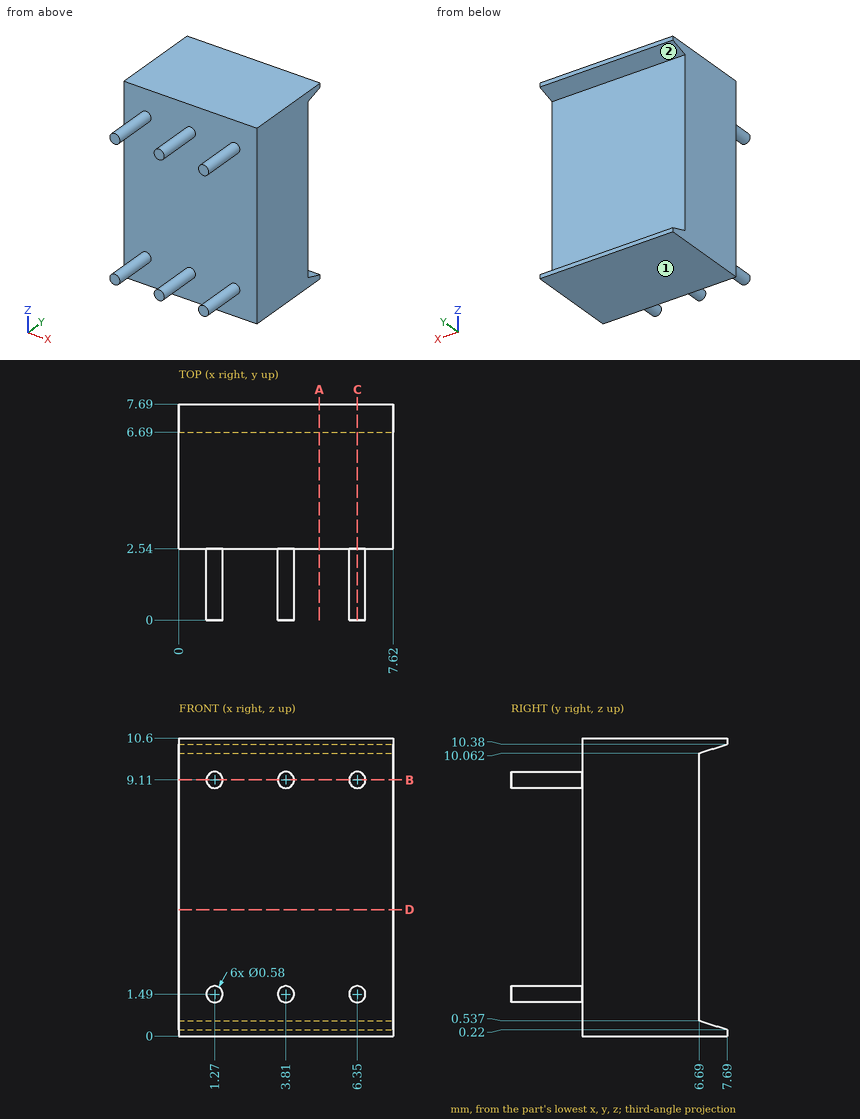
Part print with two shaded views. Sizes in mm from the minimum x, y, z corner. A direction names the side the tool comes from. Round coordinates to 2 decimals unless told otherwise and drop trailing zeros. Loops run counter-clockwise (first coordinate to the right, second up) from the corner with the lowest first, then second, coordinate; pieces in that order, holes last.
1. Slice it at A-A (x = 5). Give the cut face in (y, z).
Solutions:
outline: (2.54, 0) - (7.69, 0) - (7.69, 0.22) - (6.69, 0.54) - (6.69, 10.06) - (7.69, 10.38) - (7.69, 10.6) - (2.54, 10.6) - close
2. Drill centre lines: line 1 along Y through (x, z) = (7, 9.25); line 2 along Z through (x, y) = (4, 1.75); line 3 along Z through (x, y) = (5.75, 6.75). Where is each one in solid material? Low to high.
Solutions:
line 1: y = 2.54 to 6.69
line 2: z = 1.27 to 1.71, 8.89 to 9.33
line 3: z = 0 to 0.52, 10.08 to 10.6
3. Flat gauge pins, fed straight in: pin 1 (1 mm diameter, centred on x = 3.5, z = 8.5, fed in from -Y); pin 2 (4 mm diameter, centred on x = 5.5, z = 4.5, fed in from +Y); pin 3 (4 mm diameter, centred on x = 6, z = 4, fed in from -Y). Where does each tip first touch, or does it go through?
Solutions:
pin 1: stops at y = 0
pin 2: stops at y = 6.69
pin 3: stops at y = 2.54
4. Slice it at D-D (z = 4.5). Give the cut face in (x, y).
Solutions:
outline: (0, 2.54) - (7.62, 2.54) - (7.62, 6.69) - (0, 6.69) - close
5. Slice it at B-B (z = 9.11). Give the cut face in (x, y).
Solutions:
outline: (0, 2.54) - (0.98, 2.54) - (0.98, 0) - (1.56, 0) - (1.56, 2.54) - (3.52, 2.54) - (3.52, 0) - (4.1, 0) - (4.1, 2.54) - (6.06, 2.54) - (6.06, 0) - (6.64, 0) - (6.64, 2.54) - (7.62, 2.54) - (7.62, 6.69) - (0, 6.69) - close
6. 3-axis set-ups, long thin cutter, end or side, ignore diameter. For the marked faces 1 and 2: which of +Z, -Z, +X, -X, +Y, -Y reach the whole face in a straight line?
Solutions:
face 1: -Z, +X, -X, +Y, -Y
face 2: +X, -X, +Y
7. Slice it at C-C (x = 6.35). Give the cut face in (y, z).
Solutions:
outline: (0, 1.2) - (2.54, 1.2) - (2.54, 0) - (7.69, 0) - (7.69, 0.22) - (6.69, 0.54) - (6.69, 10.06) - (7.69, 10.38) - (7.69, 10.6) - (2.54, 10.6) - (2.54, 9.4) - (0, 9.4) - (0, 8.82) - (2.54, 8.82) - (2.54, 1.78) - (0, 1.78) - close
